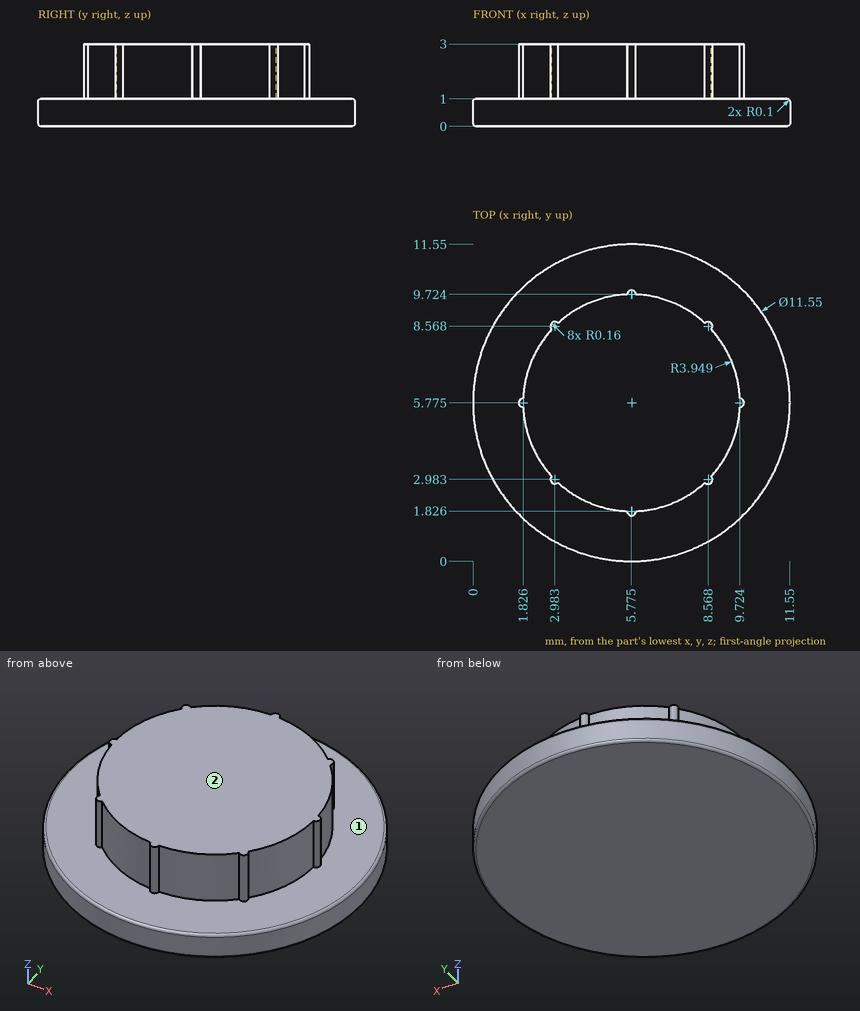
The drawing under review shows one solid part. Ordinate dimensions are in mm from its lowest x, y, z. A direction names the side the tool comes from. Give positions to 0.01 mm unless a question says otherwise; leave off trailing zeros. Answer in a Markdown table with one row per item. Add a question column.
1. To check wall thickness, follow line 1 along Z through (x, y) = (1.5, 6.5); line 2 along X through (y, z) = (9.75, 1.45) (1 decimal); line 3 along X through (y, z) = (6, 1.45). State the ranges of each line that lie inside material, in increasing order.
2. Machinability: for the marked faces 1 and 2, which of the approach directions +Z, -Z, +X, -X, +Y, -Y give a long, thin tool a straight path to every point of the face, cutting with its end or side? Answer none if there is none.
3. For pin 1 Ø2 at (x, y) = (6.5, 1.5) entering from -Z, flat-tipped, find the tip position at first contact; note if it passes through.
The answers:
| question | item | result |
|---|---|---|
| 1 | line 1 | 0 to 1 |
| 1 | line 2 | 5.6 to 5.9 |
| 1 | line 3 | 1.83 to 9.72 |
| 2 | face 1 | +Z |
| 2 | face 2 | +Z, +X, -X, +Y, -Y |
| 3 | pin 1 | z = 0 |
